```python
from build123d import *

# Parameters (mm, degrees)
SKETCH_1_R          = 1.5
EXTRUDE_1_DEPTH     = 8
CUT_EXTRUDE_1_DEPTH = 177.295206968


with BuildPart() as part:
    # 草图1 → 凸台-拉伸1 (new body)
    with BuildSketch(Plane.XY):
        with BuildLine():
            Line((5, 0), (165, 0))
            ThreePointArc((165, 0), (168.535533906, 1.464466094), (170, 5))
            Line((170, 5), (170, 11))
            Line((170, 11), (170, 16))
            Line((170, 16), (170, 46))
            Line((170, 46), (161.5, 46))
            ThreePointArc((161.5, 46), (157.964466094, 44.535533906), (156.5, 41))
            Line((156.5, 41), (156.5, 21))
            ThreePointArc((156.5, 21), (155.035533906, 17.464466094), (151.5, 16))
            Line((151.5, 16), (18.5, 16))
            ThreePointArc((18.5, 16), (14.964466094, 17.464466094), (13.5, 21))
            Line((13.5, 21), (13.5, 41))
            ThreePointArc((13.5, 41), (12.035533906, 44.535533906), (8.5, 46))
            Line((8.5, 46), (0, 46))
            Line((0, 46), (0, 16))
            Line((0, 16), (0, 11))
            Line((0, 11), (0, 5))
            ThreePointArc((0, 5), (1.464466094, 1.464466094), (5, 0))
        make_face()
        with Locations((5, 11)):
            Circle(SKETCH_1_R, mode=Mode.SUBTRACT)
        with Locations(Location((5, 5, 0), (0, 0, 180))):
            Circle(SKETCH_1_R, mode=Mode.SUBTRACT)
        with Locations((165, 5)):
            Circle(SKETCH_1_R, mode=Mode.SUBTRACT)
        with Locations(Location((165, 11, 0), (0, 0, 180))):
            Circle(SKETCH_1_R, mode=Mode.SUBTRACT)
        with Locations((6, 41)):
            Circle(SKETCH_1_R, mode=Mode.SUBTRACT)
        with Locations(Location((164, 41, 0), (0, 0, 180))):
            Circle(SKETCH_1_R, mode=Mode.SUBTRACT)
    extrude(amount=EXTRUDE_1_DEPTH)

    # 草图2 → 切除-拉伸1 (cut, through all)
    with BuildSketch(Plane.XY.offset(8)):
        with BuildLine():
            Line((-0.44, 36.7), (-0.44, 23.3))
            ThreePointArc((-0.44, 23.3), (6.26, 30), (-0.44, 36.7))
        make_face()
        with BuildLine():
            Line((170.44, 36.7), (170.44, 23.3))
            ThreePointArc((170.44, 23.3), (163.74, 30), (170.44, 36.7))
        make_face()
    extrude(amount=-CUT_EXTRUDE_1_DEPTH, mode=Mode.SUBTRACT)


solid = part.part
```
The listing builds one solid part. Answer for the finished solid, in the listing's coordinates (mm). A direction names the side the tool comes from. Give positions to 0.01 mm unless a question says otherwise; leave off trailing zeros. Write each loop counter-clockwise with the first axis right and the second up, starting at its lowest first coordinate (ties: lowest second). Pieces come first, ordered by that corner, then holes. Notation, with made-up numbers: (-14.5, -17) - (36.5, -17) arc R22 ccw to (36.5, -8) - close; hole circle Ø8 at (84, 61.5). An arc over 180 degrees is marked (long way). Use one line per item in the form item = value. Start each with the question number.
1) Find section A-A on z = 3.25. Determine the outline of the cut face in (x, y).
2) Find section B-B on y = 11. Determine the outline of the cut face in (x, z).
3) Find section C-C on y = 19. Determine the outline of the cut face in (x, z).
4) The mould has two halves that part along X. Classify faces 1 (the face through (170, 14, 4)), 2 (the face through (15, 17.43, 3.94)), 3 (the face through (1, 2, 4)): pulls with the +X half, pulls with the -X half, needs draft (parallel to the pull), parting line crosses it, or undercut.
5) Find section D-D on x = 57.5. Determine the outline of the cut face in (y, z), plus the area to 3 significant figures.
6) A tool of negligible diameter and unlimited length cuts with its end or side. For faces 4 (the face through (84, 0, 4)), 5 (the face through (156.5, 31, 4)), from which of +Z, -Z, +X, -X, +Y, -Y can it reach the whole face along a straight path? Write none if from no direction.
7) Consider line 1 along X through (y, z) = (25.5, 2.75); line 2 along X through (y, z) = (6, 5.75); line 3 along Y through (x, z) = (5, 5.5). Determine where each line is inside the solid, lowest interval first. Write a range as from..to.
8) Flat-ended cylindrical pins translate along their axes: pin 1 Ø2.5 at (x, z) = (62, 5) entering from +Y; pin 2 Ø2.5 at (x, y) = (165, 11) entering from -Z; pin 3 Ø4 at (y, z) = (31, 3.5) entering from +X. Find the tip coordinate at first contact, or state that the pin passes through.
Geometry results:
q1.outline = (0, 5) arc R5 ccw to (5, 0) - (165, 0) arc R5 ccw to (170, 5) - (170, 23.31) arc R6.7 cw to (170, 36.69) - (170, 46) - (161.5, 46) arc R5 ccw to (156.5, 41) - (156.5, 21) arc R5 cw to (151.5, 16) - (18.5, 16) arc R5 cw to (13.5, 21) - (13.5, 41) arc R5 ccw to (8.5, 46) - (0, 46) - (0, 36.69) arc R6.7 cw to (0, 23.31) - close; hole circle Ø3 at (5, 5); hole circle Ø3 at (5, 11); hole circle Ø3 at (6, 41); hole circle Ø3 at (164, 41); hole circle Ø3 at (165, 5); hole circle Ø3 at (165, 11)
q2.outline = (0, 0) - (3.5, 0) - (3.5, 8) - (0, 8) - close; (6.5, 0) - (163.5, 0) - (163.5, 8) - (6.5, 8) - close; (166.5, 0) - (170, 0) - (170, 8) - (166.5, 8) - close
q3.outline = (0, 0) - (13.92, 0) - (13.92, 8) - (0, 8) - close; (156.08, 0) - (170, 0) - (170, 8) - (156.08, 8) - close
q4.face_1 = pulls with the +X half
q4.face_2 = undercut
q4.face_3 = pulls with the -X half
q5.outline = (0, 0) - (16, 0) - (16, 8) - (0, 8) - close
q5.area = 128 mm2
q6.face_4 = +Z, -Z, +X, -X, -Y
q6.face_5 = +Z, -Z, +Y
q7.line_1 = 4.52..13.5, 156.5..165.48
q7.line_2 = 0..3.88, 6.12..163.88, 166.12..170
q7.line_3 = 0..3.5, 6.5..9.5, 12.5..26.09, 33.91..39.88, 42.12..46
q8.pin_1 = 16
q8.pin_2 = through
q8.pin_3 = 164.45
